Can you work these out from the model? Positions are in its coordinate system, mm. A direction names the side the tool comes from. Give positions to 0.01 mm unless a question says otherwise; leave off trailing zeros. Order: outer loops, then holes, each group sorted by start corner. A loop starts at its lowest first (then second) coordinate and runs counter-clockwise, first axis right, second up. Notation, with made-up numbers: (67, -40) - (120, -40) arc R31 cw to (120, -15) - close; hole circle Ø3 at (-31.5, 6). An arc over 180 degrees is marked (long way). Use one line per item in the form item = value. Start each with the question number.
1) We'd pull the mould along Y, two halves only. Please class faces 1 (the flat face through (49.944, 97.535, 9.507)), 2 (the flat face through (70.5, 7.4, 67.5)): released by +Y, released by -Y, zero draft, split by the parting line, or undercut.
2) Suppose I cut it at C-C, the plane z = -40. Write out the boundary of the cut face in (x, y).
3) Which directions (+Z, -Z, +X, -X, +Y, -Y) give clear straight access to the entire face, cutting with the end or side of a thin tool? Please do faces 3 (the flat face through (65, 57, 0)), 4 (the flat face through (38.82, 40, 1)), 5 (the flat face through (57.5, 3, -62)), 6 (the flat face through (42.5, 41, -22)).
4) For pin 1 (3 mm diameter, centred on y = 12.5, z = 29, fed in from +X); pin 2 (2.5 mm diameter, centred on x = 69, z = -69, fed in from +Y); pin 3 (6 mm diameter, centred on x = 3.5, z = 19, fed in from +Y), each with a flat end and sliding along its axis, tell me the tip position at first contact or that it passes through.
5) Please list where these lines run through material, in increasing order: probe 1 along X at (y, z) = (83, -50); probe 2 along X at (y, z) = (11, -58); probe 3 along Y at (x, z) = (20, -58).
6) Suppose I cut it at B-B, the plane x = 60. State how many separate pieces and enclosed holes the cut face has, and give its area (3 significant figures).
7) Suppose I cut it at A-A, the plane y = 38.5. Write out the boundary of the cut face in (x, z).
```python
from build123d import *

# Parameters (mm, degrees)
SKETCH1_W                                 = 80
SKETCH1_H                                 = 60
BOSS_EXTRUDE1_DEPTH                       = 100
CUT_EXTRUDE1_START                        = 5
SKETCH2_W                                 = 35
SKETCH2_H                                 = 55
CUT_EXTRUDE1_DEPTH                        = 95
SKETCH3_W                                 = 80
SKETCH3_H                                 = 5
BOSS_EXTRUDE2_DEPTH                       = 70
BOSS_EXTRUDE3_DEPTH                       = 10
SKETCH5_W                                 = 20
SKETCH5_H                                 = 2.5
CUT_EXTRUDE2_DEPTH                        = 7.5
SKETCH6_W                                 = 35
SKETCH6_H                                 = 12
CUT_EXTRUDE4_DEPTH                        = 57.5
CUT_EXTRUDE6_REACH                        = 184.483
SKETCH7_R                                 = 4
SKETCH9_W                                 = 80
SKETCH9_H                                 = 50
BOSS_EXTRUDE4_DEPTH                       = 5
SKETCH13_W                                = 8
SKETCH13_H                                = 7
CUT_EXTRUDE8_BUTTON_HOLES_DEPTH           = 166.90660023
BOSS_EXTRUDE5_OLED_MOUNT_DEPTH            = 10
BOSS_EXTRUDE6_OLED_MOUNT_DEPTH            = 1
BOSS_EXTRUDE7_START                       = -2.5
BOSS_EXTRUDE7_OLED_MOUNT_DEPTH            = 1
BOSS_EXTRUDE8_OLED_MOUNT_DEPTH            = 1
BOSS_EXTRUDE13_OLED_MOUNT_SUPPORT_DEPTH   = 30
CUT_EXTRUDE9_OLED_CABLE_DEPTH             = 10
CUT_EXTRUDE9_OLED_CABLE_DEPTH_BACK        = 154.430766146
SKETCH18_W                                = 2.36
SKETCH18_H                                = 8
BOSS_EXTRUDE12_OLED_CABLE_GUIDE_REACH     = 162.39
SKETCH20_W                                = 5
SKETCH20_H                                = 5
CUT_EXTRUDE10_SOLENOID_WIRE_HOLE_DEPTH    = 166.90660023
SKETCH21_W                                = 5
SKETCH21_H                                = 32
BOSS_EXTRUDE9_SOLENOID_SIDE_SUPPORT_DEPTH = 13
CHAMFER3_THUMB_SIZE                       = 2.5
CHAMFER5_THUMB_SIZE                       = 4.5
CHAMFER5_THUMB_SIZE2                      = 7.794228634
CHAMFER5_THUMB_PART_2_SIZE                = 4.5
CHAMFER5_THUMB_PART_2_SIZE2               = 7.794228634
CHAMFER5_THUMB_PART_3_SIZE                = 4.5
CHAMFER5_THUMB_PART_3_SIZE2               = 7.794228634
BOSS_EXTRUDE5_GUIDE_DEPTH                 = 180
SKETCH49_W                                = 5
SKETCH49_H                                = 5
BOSS_EXTRUDE14_DEPTH                      = 5
CHAMFER8_SIZE                             = 5


with BuildPart() as part:
    # Sketch1 → Boss-Extrude1 (new body)
    with BuildSketch(Plane(origin=(0, 0, 0), x_dir=(1, 0, 0), z_dir=(0, 1, 0))):
        with Locations((40, 30)):
            Rectangle(SKETCH1_W, SKETCH1_H)
    extrude(amount=BOSS_EXTRUDE1_DEPTH)

    # Sketch2 → Cut-Extrude1 (cut)
    with BuildSketch(Plane(origin=(0, 0, 0), x_dir=(1, 0, 0), z_dir=(0, 1, 0)).offset(CUT_EXTRUDE1_START)):
        with Locations((20, 30)):
            Rectangle(SKETCH2_W, SKETCH2_H)
        with Locations((60, 30)):
            Rectangle(SKETCH2_W, SKETCH2_H)
    extrude(amount=CUT_EXTRUDE1_DEPTH, mode=Mode.SUBTRACT)

    # Sketch3 → Boss-Extrude2 (add)
    with BuildSketch(Plane.XY):
        with Locations((40, 2.5)):
            Rectangle(SKETCH3_W, SKETCH3_H)
    extrude(amount=BOSS_EXTRUDE2_DEPTH)

    # Sketch4 → Boss-Extrude3 (add)
    with BuildSketch(Plane(origin=(0, 5, 0), x_dir=(1, 0, 0), z_dir=(0, 1, 0))):
        Polygon((80, 0), (77.5, 0), (77.5, -67.5), (42.5, -67.5), (42.5, 0), (37.5, 0), (37.5, -67.5), (2.5, -67.5), (2.5, 0), (0, 0), (0, -70), (80, -70), align=None)
    extrude(amount=BOSS_EXTRUDE3_DEPTH)

    # Sketch5 → Cut-Extrude2 (cut)
    with BuildSketch(Plane(origin=(0, 15, 0), x_dir=(1, 0, 0), z_dir=(0, 1, 0))):
        with Locations((20, -68.75)):
            Rectangle(SKETCH5_W, SKETCH5_H)
        with Locations((60, -68.75)):
            Rectangle(SKETCH5_W, SKETCH5_H)
    extrude(amount=-CUT_EXTRUDE2_DEPTH, mode=Mode.SUBTRACT)

    # Sketch6 → Cut-Extrude4 (cut)
    with BuildSketch(Plane.XY):
        with Locations((20, 11)):
            Rectangle(SKETCH6_W, SKETCH6_H)
        with Locations((60, 11)):
            Rectangle(SKETCH6_W, SKETCH6_H)
    extrude(amount=-CUT_EXTRUDE4_DEPTH, mode=Mode.SUBTRACT)

    # Sketch7 → Cut-Extrude6 (cut, up to next)
    with BuildSketch(Plane(origin=(0, 0, -60), x_dir=(-1, 0, 0), z_dir=(0, 0, -1)), mode=Mode.PRIVATE) as cut_extrude6_sk1:
        with Locations((-20, 11.5)):
            Circle(SKETCH7_R)
    cut_extrude6_tool1 = extrude(cut_extrude6_sk1.sketch, amount=-CUT_EXTRUDE6_REACH, mode=Mode.PRIVATE) & part.part
    # Sketch7 → Cut-Extrude6 (cut, up to next)
    with BuildSketch(Plane(origin=(0, 0, -60), x_dir=(-1, 0, 0), z_dir=(0, 0, -1)), mode=Mode.PRIVATE) as cut_extrude6_sk2:
        with Locations((-60, 11.5)):
            Circle(SKETCH7_R)
    cut_extrude6_tool2 = extrude(cut_extrude6_sk2.sketch, amount=-CUT_EXTRUDE6_REACH, mode=Mode.PRIVATE) & part.part
    add(cut_extrude6_tool1.solids().sort_by_distance((20, 11.5, -60))[0], mode=Mode.SUBTRACT)
    add(cut_extrude6_tool2.solids().sort_by_distance((60, 11.5, -60))[0], mode=Mode.SUBTRACT)

    # Sketch9 → Boss-Extrude4 (add)
    with BuildSketch(Plane(origin=(0, 0, 0), x_dir=(1, 0, 0), z_dir=(0, 1, 0))):
        with Locations((40, 85)):
            Rectangle(SKETCH9_W, SKETCH9_H)
    extrude(amount=BOSS_EXTRUDE4_DEPTH)

    # Sketch13 → Cut-Extrude8 (Button Holes) (cut, through all)
    with BuildSketch(Plane(origin=(0, 5, 0), x_dir=(1, 0, 0), z_dir=(0, 1, 0))):
        with Locations((20, -61)):
            Rectangle(SKETCH13_W, SKETCH13_H)
        with Locations((60, -61)):
            Rectangle(SKETCH13_W, SKETCH13_H)
    extrude(amount=-CUT_EXTRUDE8_BUTTON_HOLES_DEPTH, mode=Mode.SUBTRACT)

    # Sketch14 → Boss-Extrude5 (OLED Mount) (add)
    with BuildSketch(Plane.XY):
        Polygon((25, 100), (26, 100), (26, 71), (54, 71), (54, 100), (55, 100), (55, 70), (54, 70), (26, 70), (25, 70), align=None)
    extrude(amount=BOSS_EXTRUDE5_OLED_MOUNT_DEPTH)

    # Sketch15 → Boss-Extrude6 (OLED Mount) (add)
    with BuildSketch(Plane.XY.offset(10)):
        Polygon((26, 71), (34, 71), (26, 75), align=None)
        Polygon((54, 75), (54, 71), (46, 71), align=None)
    extrude(amount=-BOSS_EXTRUDE6_OLED_MOUNT_DEPTH)

    # Sketch15<2> → Boss-Extrude7 (OLED Mount) (add)
    with BuildSketch(Plane.XY.offset(10).offset(BOSS_EXTRUDE7_START)):
        Polygon((26, 71), (34, 71), (26, 75), align=None)
        Polygon((54, 75), (54, 71), (46, 71), align=None)
    extrude(amount=-BOSS_EXTRUDE7_OLED_MOUNT_DEPTH)

    # Sketch17 → Boss-Extrude8 (OLED Mount) (add)
    with BuildSketch(Plane.XY.offset(10)):
        Polygon((54, 95), (54, 100), (46, 100), align=None)
        Polygon((26, 100), (34, 100), (26, 95), align=None)
    extrude(amount=-BOSS_EXTRUDE8_OLED_MOUNT_DEPTH)

    # Sketch32 → Boss-Extrude13 OLED Mount Support) (add)
    with BuildSketch(Plane.ZY.offset(-25)):
        Polygon((0, 70), (10, 70), (0, 60), align=None)
    extrude(amount=-BOSS_EXTRUDE13_OLED_MOUNT_SUPPORT_DEPTH)

    # Sketch18 → Cut-Extrude9 (OLED Cable) (cut, two sides: drawn at the far end of the back side and taken through both)
    with BuildSketch(Plane(origin=(0, 71, 0), x_dir=(1, 0, 0), z_dir=(0, 1, 0)).offset(-CUT_EXTRUDE9_OLED_CABLE_DEPTH_BACK)):
        with Locations((40, -1)):
            Rectangle(SKETCH18_W, SKETCH18_H)
    extrude(amount=CUT_EXTRUDE9_OLED_CABLE_DEPTH + CUT_EXTRUDE9_OLED_CABLE_DEPTH_BACK, mode=Mode.SUBTRACT)

    # Boss-Extrude12 (OLED Cable Guide): up to this plane
    boss_extrude12_oled_cable_guide_end = Plane(origin=(55, 70, 10), z_dir=(0, -0.7071067811865477, 0.7071067811865474))
    # Sketch31 → Boss-Extrude12 (OLED Cable Guide) (add, up to the surface)
    with BuildSketch(Plane(origin=(0, 15, 0), x_dir=(1, 0, 0), z_dir=(0, 1, 0)), mode=Mode.PRIVATE) as boss_extrude12_oled_cable_guide_sk1:
        Polygon((37.5, 0), (38.82, 0), (38.82, -5), (41.18, -5), (41.18, 0), (42.5, 0), (42.5, -7), (37.5, -7), align=None)
    boss_extrude12_oled_cable_guide_tool1 = split(extrude(boss_extrude12_oled_cable_guide_sk1.sketch, amount=BOSS_EXTRUDE12_OLED_CABLE_GUIDE_REACH, mode=Mode.PRIVATE), bisect_by=boss_extrude12_oled_cable_guide_end, keep=Keep.BOTH, mode=Mode.PRIVATE)
    add(boss_extrude12_oled_cable_guide_tool1.solids().sort_by_distance((38.16, 15, 0.086023))[0])

    # Sketch20 → Cut-Extrude10 (Solenoid Wire Hole) (cut, through all)
    with BuildSketch(Plane(origin=(0, 5, 0), x_dir=(1, 0, 0), z_dir=(0, 1, 0))):
        with Locations((60, 62.5)):
            Rectangle(SKETCH20_W, SKETCH20_H)
        with Locations((20, 62.5)):
            Rectangle(SKETCH20_W, SKETCH20_H)
    extrude(amount=-CUT_EXTRUDE10_SOLENOID_WIRE_HOLE_DEPTH, mode=Mode.SUBTRACT)

    # Sketch21 → Boss-Extrude9 (Solenoid Side Support) (add)
    with BuildSketch(Plane(origin=(0, 5, 0), x_dir=(1, 0, 0), z_dir=(0, 1, 0))):
        with Locations((70, 76)):
            Rectangle(SKETCH21_W, SKETCH21_H)
        with Locations((50, 76)):
            Rectangle(SKETCH21_W, SKETCH21_H)
        with Locations((30, 76)):
            Rectangle(SKETCH21_W, SKETCH21_H)
        with Locations((10, 76)):
            Rectangle(SKETCH21_W, SKETCH21_H)
    extrude(amount=BOSS_EXTRUDE9_SOLENOID_SIDE_SUPPORT_DEPTH)

    # Chamfer3 (Thumb)
    chamfer3_thumb_edges = [part.edges().sort_by_distance(p)[0] for p in [
        (20, 7.5, 67.5),
        (60, 7.5, 67.5),
    ]]
    chamfer(chamfer3_thumb_edges, length=CHAMFER3_THUMB_SIZE - 0.0001)  # a hair under: the kernel refuses the full size

    # Chamfer5 (Thumb)
    chamfer5_thumb_edges = [part.edges().sort_by_distance(p)[0] for p in [
        (70, 15, 68.75),
    ]]
    chamfer5_thumb_side = [part.faces().sort_by_distance(p)[0] for p in [
        (78.266129032, 15, 38.266129032),
    ]]
    chamfer(chamfer5_thumb_edges, length=CHAMFER5_THUMB_SIZE, length2=CHAMFER5_THUMB_SIZE2, reference=chamfer5_thumb_side[0])

    # Chamfer5 (Thumb) part 2
    chamfer5_thumb_part_2_edges = [part.edges().sort_by_distance(p)[0] for p in [
        (50, 15, 68.75),
        (30, 15, 68.75),
    ]]
    chamfer5_thumb_part_2_side = [part.faces().sort_by_distance(p)[0] for p in [
        (40, 15, 41.718085106),
    ]]
    chamfer(chamfer5_thumb_part_2_edges, length=CHAMFER5_THUMB_PART_2_SIZE, length2=CHAMFER5_THUMB_PART_2_SIZE2, reference=chamfer5_thumb_part_2_side[0])

    # Chamfer5 (Thumb) part 3
    chamfer5_thumb_part_3_edges = [part.edges().sort_by_distance(p)[0] for p in [
        (10, 15, 68.75),
    ]]
    chamfer5_thumb_part_3_side = [part.faces().sort_by_distance(p)[0] for p in [
        (1.733870968, 15, 38.266129032),
    ]]
    chamfer(chamfer5_thumb_part_3_edges, length=CHAMFER5_THUMB_PART_3_SIZE, length2=CHAMFER5_THUMB_PART_3_SIZE2, reference=chamfer5_thumb_part_3_side[0])

    # Sketch37 → Boss-Extrude5 (Guide) (add, through all)
    with BuildSketch(Plane.XY.offset(70)):
        Polygon((80, 0), (83, 0), (80, 3), align=None)
        Polygon((0, 0), (-3, 0), (0, 3), align=None)
    extrude(amount=-BOSS_EXTRUDE5_GUIDE_DEPTH)

    # Sketch49 → Boss-Extrude14 (add)
    with BuildSketch(Plane(origin=(0, 15, 0), x_dir=(1, 0, 0), z_dir=(0, 1, 0))):
        with Locations((40, -9.5)):
            Rectangle(SKETCH49_W, SKETCH49_H)
    extrude(amount=BOSS_EXTRUDE14_DEPTH)

    # Chamfer8
    chamfer8_edges = [part.edges().sort_by_distance(p)[0] for p in [
        (40, 20, 12),
    ]]
    chamfer(chamfer8_edges, length=CHAMFER8_SIZE - 0.0001)  # a hair under: the kernel refuses the full size


solid = part.part
```
Result sheet:
q1.face_1 = undercut
q1.face_2 = zero draft
q2.outline = (-3, 0) - (83, 0) - (80, 3) - (80, 100) - (77.5, 100) - (77.5, 5) - (42.5, 5) - (42.5, 100) - (37.5, 100) - (37.5, 5) - (2.5, 5) - (2.5, 100) - (0, 100) - (0, 3) - close
q3.face_3 = +Z, +X
q3.face_4 = -Y
q3.face_5 = +Y, -Y
q3.face_6 = none
q4.pin_1 = 80
q4.pin_2 = 18
q4.pin_3 = 15
q5.probe_1 = 0 to 2.5, 37.5 to 42.5, 77.5 to 80
q5.probe_2 = 0 to 16.03, 23.97 to 56.03, 63.97 to 80
q5.probe_3 = 0 to 7.5, 15.5 to 100
q6.separate_pieces = 5
q6.enclosed_holes = 0
q6.area = 1,270 mm²
q7.outline = (0, -60) - (80, -60) - (80, 0) - (42.5, 0) - (42.5, 7) - (37.5, 7) - (37.5, 0) - (0, 0) - close; hole (2.5, -57.5) - (37.5, -57.5) - (37.5, -2.5) - (2.5, -2.5) - close; hole (38.82, -3) - (41.18, -3) - (41.18, 5) - (38.82, 5) - close; hole (42.5, -57.5) - (77.5, -57.5) - (77.5, -2.5) - (42.5, -2.5) - close
